from build123d import *

# Parameters (mm, degrees)
BASE_FLANGE1_DEPTH      = 15
BASE_FLANGE1_DEPTH_BACK = 15
SKETCH6_R               = 3.175
CUT_EXTRUDE1_DEPTH      = 53.665358634
SKETCH7_R               = 1.984375
CUT_EXTRUDE2_DEPTH      = 10


# Sheet-metal steps are written as plain solids
with BuildPart() as part:
    # Sketch1 → Base-Flange1 (new, two sides: drawn at the far end of the back side and taken through both)
    with BuildSketch(Plane.XY.offset(-BASE_FLANGE1_DEPTH_BACK)):
        with BuildLine():
            Line((-40, 0), (-22, 0))
            ThreePointArc((-22, 0), (-20.585786438, 0.585786438), (-20, 2))
            Line((-20, 2), (-20, 27.2))
            ThreePointArc((-20, 27.2), (-19.179898987, 29.179898987), (-17.2, 30))
            Line((-17.2, 30), (17.2, 30))
            ThreePointArc((17.2, 30), (19.179898987, 29.179898987), (20, 27.2))
            Line((20, 27.2), (20, 2))
            ThreePointArc((20, 2), (20.585786438, 0.585786438), (22, 0))
            Line((22, 0), (40, 0))
            Line((40, 0), (40, -0.8))
            Line((40, -0.8), (22, -0.8))
            ThreePointArc((22, -0.8), (20.020101013, 0.020101013), (19.2, 2))
            Line((19.2, 2), (19.2, 27.2))
            ThreePointArc((19.2, 27.2), (18.614213562, 28.614213562), (17.2, 29.2))
            Line((17.2, 29.2), (-17.2, 29.2))
            ThreePointArc((-17.2, 29.2), (-18.614213562, 28.614213562), (-19.2, 27.2))
            Line((-19.2, 27.2), (-19.2, 2))
            ThreePointArc((-19.2, 2), (-20.020101013, 0.020101013), (-22, -0.8))
            Line((-22, -0.8), (-40, -0.8))
            Line((-40, -0.8), (-40, 0))
        make_face()
    extrude(amount=BASE_FLANGE1_DEPTH + BASE_FLANGE1_DEPTH_BACK)

    # Sketch6 → Cut-Extrude1 (cut, through all)
    with BuildSketch(Plane(origin=(0, 30, 0), x_dir=(1, 0, 0), z_dir=(0, 1, 0))):
        with Locations(Location((0, 0, 0), (0, 0, 270))):
            Circle(SKETCH6_R)
    extrude(amount=-CUT_EXTRUDE1_DEPTH, mode=Mode.SUBTRACT)

    # Sketch7 → Cut-Extrude2 (cut)
    with BuildSketch(Plane(origin=(0, 0, 0), x_dir=(1, 0, 0), z_dir=(0, 1, 0))):
        with Locations(Location((30, -6, 0), (0, 0, 180))):
            Circle(SKETCH7_R)
        with Locations(Location((30, 6, 0), (0, 0, 180))):
            Circle(SKETCH7_R)
        with Locations(Location((-30.742868113, 6, 0), (0, 0, 180))):
            Circle(SKETCH7_R)
        with Locations(Location((-30.742868113, -6, 0), (0, 0, 180))):
            Circle(SKETCH7_R)
    extrude(amount=-CUT_EXTRUDE2_DEPTH, mode=Mode.SUBTRACT)


solid = part.part
Work out the finished part from the listing and answer in its coordinate system (mm). A direction names the side the tool comes from. Give positions to 0.01 mm unless a question says otherwise; leave off trailing zeros. Write each loop counter-clockwise with the first axis right and the second up, starting at its lowest first coordinate (ties: lowest second). Pieces come first, ordered by that corner, then holes. Notation, with made-up numbers: (16, -8) - (36, -8) arc R11 ccw to (36, 3) - close; hole circle Ø4 at (85, -23.5). An arc over 180 degrees is marked (long way). One line per item, written item: value. Start each with the question number.
1. Find section B-B (z = 6). Write down the section's boundary in (x, y).
2. Find section A-A (x = 30). Write down the section's boundary in (y, z).
3. For a pull along Z with two mould halves and no side action, classify faces 1 (the flat face through (31, 0, 0)), 2 (the cylindrical face through (-28.76, -0.39, -5.91)), 3 (the flat face through (0.2, 29.5, 15)) as +Z half, -Z half, draft (parallel to the pull), parting line (faces both ways), or undercut.
4. Find section C-C (y = 10). Write down the section's boundary in (x, z).
5. Consider probe 1 along X at (y, z) = (18, -12); probe 2 along Z at (x, y) = (30, -0.2); probe 3 along Y at (x, z) = (23.5, 13.75). Determine where each line is inside the solid, lowest interval first.
6. For faces 4 (the flat face through (20, 15, 0)), 5 (the flat face through (-31, 0, 0)), 6 (the cylindrical face through (-20, 0.04, -0.21)), determine the directions among +Z, -Z, +X, -X, +Y, -Y from which every point of the face is accessible in a straight line to the end or side of a thin tool.
7. Given pin 1 (9 mm diameter, centred on x = 31.5, z = -4.5, fed in from +Y); pin 2 (2 mm diameter, centred on y = 24, z = -2, fed in from -X); pin 3 (5 mm diameter, centred on y = 8.5, z = -9.5, fed in from +X), each flat-ended and moving along its own axis, determine where each tip first touches the part or whether it passes through.
8. Find section D-D (z = 0). Write down the section's boundary in (x, y) (3 decimals).
Geometry results:
1. outline: (-40, -0.8) - (-32.73, -0.8) - (-32.73, 0) - (-40, 0) - close; (-28.76, -0.8) - (-22, -0.8) arc R2.8 ccw to (-19.2, 2) - (-19.2, 27.2) arc R2 cw to (-17.2, 29.2) - (17.2, 29.2) arc R2 cw to (19.2, 27.2) - (19.2, 2) arc R2.8 ccw to (22, -0.8) - (28.02, -0.8) - (28.02, 0) - (22, 0) arc R2 cw to (20, 2) - (20, 27.2) arc R2.8 ccw to (17.2, 30) - (-17.2, 30) arc R2.8 ccw to (-20, 27.2) - (-20, 2) arc R2 cw to (-22, 0) - (-28.76, 0) - close; (31.98, -0.8) - (40, -0.8) - (40, 0) - (31.98, 0) - close
2. outline: (-0.8, -15) - (0, -15) - (0, -7.98) - (-0.8, -7.98) - close; (-0.8, -4.02) - (0, -4.02) - (0, 4.02) - (-0.8, 4.02) - close; (-0.8, 7.98) - (0, 7.98) - (0, 15) - (-0.8, 15) - close
3. face 1: draft
3. face 2: undercut
3. face 3: +Z half
4. outline: (-20, -15) - (-19.2, -15) - (-19.2, 15) - (-20, 15) - close; (19.2, -15) - (20, -15) - (20, 15) - (19.2, 15) - close
5. probe 1: -20 to -19.2, 19.2 to 20
5. probe 2: -15 to -7.98, -4.02 to 4.02, 7.98 to 15
5. probe 3: -0.8 to 0
6. face 4: +Z, -Z, +X, +Y
6. face 5: +Z, -Z, -X, +Y
6. face 6: +Z, -Z, -Y
7. pin 1: y = 0
7. pin 2: x = -20
7. pin 3: x = 20
8. outline: (-40, -0.8) - (-22, -0.8) arc R2.8 ccw to (-19.2, 2) - (-19.2, 27.2) arc R2 cw to (-17.2, 29.2) - (-3.175, 29.2) - (-3.175, 30) - (-17.2, 30) arc R2.8 ccw to (-20, 27.2) - (-20, 2) arc R2 cw to (-22, 0) - (-40, 0) - close; (3.175, 29.2) - (17.2, 29.2) arc R2 cw to (19.2, 27.2) - (19.2, 2) arc R2.8 ccw to (22, -0.8) - (40, -0.8) - (40, 0) - (22, 0) arc R2 cw to (20, 2) - (20, 27.2) arc R2.8 ccw to (17.2, 30) - (3.175, 30) - close
